```python
from build123d import *

# Parameters (mm, degrees)
F0_W     = 10
F0_H     = 10
F1_DEPTH = 2
F3_DEPTH = 1


with BuildPart() as f1:
    # F0 (on Top) → F1 (new body)
    with BuildSketch(Plane.XY):
        Rectangle(F0_W, F0_H)
    extrude(amount=F1_DEPTH)

    # F2 (on face) → F3 (cut)
    with BuildSketch(Plane(origin=(0, 0, 0), x_dir=(1, 0, 0), z_dir=(0, 0, -1))):
        with BuildLine():
            ThreePointArc((-0.5, 3.8660254038), (-0.5, 2.1339745962), (1, 3))
            ThreePointArc((1, 3), (0.8660254038, 3.5), (0.5, 3.8660254038))
            Line((0.5, 3.8660254038), (0.5, 3))
            Line((0.5, 3), (-0.5, 3))
            Line((-0.5, 3), (-0.5, 3.8660254038))
        make_face()
        with BuildLine():
            Line((0.5, 3), (0.5, 3.8660254038))
            ThreePointArc((0.5, 3.8660254038), (0, 4), (-0.5, 3.8660254038))
            Line((-0.5, 3.8660254038), (-0.5, 3))
            Line((-0.5, 3), (0.5, 3))
        make_face()
        with BuildLine():
            ThreePointArc((-0.5, 3.8660254038), (0, 4), (0.5, 3.8660254038))
            Line((0.5, 3.8660254038), (0.5, 5))
            Line((0.5, 5), (-0.5, 5))
            Line((-0.5, 5), (-0.5, 3.8660254038))
        make_face()
        with BuildLine():
            ThreePointArc((3.8660254038, -0.5), (3.9659258263, -0.2588190451), (4, 0))
            ThreePointArc((4, 0), (3.9659258263, 0.2588190451), (3.8660254038, 0.5))
            Line((3.8660254038, 0.5), (3, 0.5))
            Line((3, 0.5), (3, -0.5))
            Line((3, -0.5), (3.8660254038, -0.5))
        make_face()
        with BuildLine():
            ThreePointArc((3.8660254038, 0.5), (3.9659258263, 0.2588190451), (4, 0))
            ThreePointArc((4, 0), (3.9659258263, -0.2588190451), (3.8660254038, -0.5))
            Line((3.8660254038, -0.5), (5, -0.5))
            Line((5, -0.5), (5, 0.5))
            Line((5, 0.5), (3.8660254038, 0.5))
        make_face()
        with BuildLine():
            Line((3, 0.5), (3.8660254038, 0.5))
            ThreePointArc((3.8660254038, 0.5), (2, 0), (3.8660254038, -0.5))
            Line((3.8660254038, -0.5), (3, -0.5))
            Line((3, -0.5), (3, 0.5))
        make_face()
        with BuildLine():
            ThreePointArc((0.5, -3.8660254038), (0.8660254038, -3.5), (1, -3))
            ThreePointArc((1, -3), (-0.5, -2.1339745962), (-0.5, -3.8660254038))
            Line((-0.5, -3.8660254038), (-0.5, -3))
            Line((-0.5, -3), (0.5, -3))
            Line((0.5, -3), (0.5, -3.8660254038))
        make_face()
        with BuildLine():
            Line((-0.5, -3), (-0.5, -3.8660254038))
            ThreePointArc((-0.5, -3.8660254038), (0, -4), (0.5, -3.8660254038))
            Line((0.5, -3.8660254038), (0.5, -3))
            Line((0.5, -3), (-0.5, -3))
        make_face()
        with BuildLine():
            ThreePointArc((0.5, -3.8660254038), (0, -4), (-0.5, -3.8660254038))
            Line((-0.5, -3.8660254038), (-0.5, -5))
            Line((-0.5, -5), (0.5, -5))
            Line((0.5, -5), (0.5, -3.8660254038))
        make_face()
        with BuildLine():
            ThreePointArc((-3.8660254038, -0.5), (-2.7411809549, -0.9659258263), (-2, 0))
            ThreePointArc((-2, 0), (-2.7411809549, 0.9659258263), (-3.8660254038, 0.5))
            Line((-3.8660254038, 0.5), (-3, 0.5))
            Line((-3, 0.5), (-3, -0.5))
            Line((-3, -0.5), (-3.8660254038, -0.5))
        make_face()
        with BuildLine():
            Line((-3, 0.5), (-3.8660254038, 0.5))
            ThreePointArc((-3.8660254038, 0.5), (-4, 0), (-3.8660254038, -0.5))
            Line((-3.8660254038, -0.5), (-3, -0.5))
            Line((-3, -0.5), (-3, 0.5))
        make_face()
        with BuildLine():
            ThreePointArc((-3.8660254038, -0.5), (-4, 0), (-3.8660254038, 0.5))
            Line((-3.8660254038, 0.5), (-5, 0.5))
            Line((-5, 0.5), (-5, -0.5))
            Line((-5, -0.5), (-3.8660254038, -0.5))
        make_face()
    extrude(amount=-F3_DEPTH, mode=Mode.SUBTRACT)


solid = f1.part
```
Work out the finished part from the listing and answer in its coordinate system (mm). A direction names the side the tool comes from. Round coordinates to 2 decimals unless told otherwise and drop trailing zeros. Write each loop counter-clockwise with the first axis right and the second up, starting at its lowest first coordinate (ties: lowest second). Pieces come first, ordered by that corner, then holes. Notation, with made-up numbers: (48, -17) -> (57, -17) arc R29 cw to (57, 5) -> close; hole circle Ø9 at (28, 83). An arc over 180 degrees is marked (long way). Write each question's results on one line, items separated by ' | '.
1) The part is cut by section C-C (x = 3). Write down the section's boundary in (y, z).
Findings:
outline: (-5, 0) -> (-1, 0) -> (-1, 1) -> (1, 1) -> (1, 0) -> (5, 0) -> (5, 2) -> (-5, 2) -> close
2) The part is cut by section A-A (z = 0.75). Write down the section's boundary in (x, y).
Findings:
outline: (-5, -5) -> (-0.5, -5) -> (-0.5, -3.87) arc R1 cw (long way) to (0.5, -3.87) -> (0.5, -5) -> (5, -5) -> (5, -0.5) -> (3.87, -0.5) arc R1 cw (long way) to (3.87, 0.5) -> (5, 0.5) -> (5, 5) -> (0.5, 5) -> (0.5, 3.87) arc R1 cw (long way) to (-0.5, 3.87) -> (-0.5, 5) -> (-5, 5) -> (-5, 0.5) -> (-3.87, 0.5) arc R1 cw (long way) to (-3.87, -0.5) -> (-5, -0.5) -> close
3) Consider line 1 along Y through (x, z) = (-4.5, 0.1); line 2 along Y through (x, z) = (0, 0.65); line 3 along Y through (x, z) = (3.75, 0.65). Determine where each line is inside the solid, lowest interval first. Write a range as [from, to].
Findings:
line 1: y = [-5, -0.5], [0.5, 5] | line 2: y = [-2, 2] | line 3: y = [-5, -0.66], [0.66, 5]
4) Which of the six approach directions +Z, -Z, +X, -X, +Y, -Y give full straight-line access (tool end or side, diameter ignored) to faces 1 (the flat face through (3, 0, 1)), 2 (the flat face through (0.5, 4.4, 0.5)), 3 (the flat face through (-4.4, -0.5, 0.5))?
Findings:
face 1: -Z | face 2: -Z, +Y | face 3: -Z, -X
5) For a pull along X with two mould halves and no side action, classify faces 4 (the cylindrical face through (2, 0, 0.5)), 5 (the flat face through (5, -0.1, 1.2)), 6 (the flat face through (0, -4, 1)), 7 (the flat face through (0, 0, 2)) as +X half, -X half, draft (parallel to the pull), parting line (faces both ways), or undercut.
Findings:
face 4: undercut | face 5: +X half | face 6: undercut | face 7: draft
6) A flat-ended cylindrical pin translates along its axis: pin 1 (1 mm diameter, centred on x = 0, y = 3, fed in from -Z). Find the tip coordinate at first contact, or state that the pin passes through.
Findings:
pin 1: stops at z = 1
7) The part is cut by section B-B (y = 4.5). Write down the section's boundary in (x, z).
Findings:
outline: (-5, 0) -> (-0.5, 0) -> (-0.5, 1) -> (0.5, 1) -> (0.5, 0) -> (5, 0) -> (5, 2) -> (-5, 2) -> close
